Answer from the drawing. Dimensions are ordinates in mm from the lowest x, y and z of the part. A direction names the side the tool comes from. Round coordinates to 2 decimals unless told otherwise and drop trailing zeros. Write each loop counter-clockwise with the first axis right and the second up, starting at its lowest first coordinate (ties: lowest second). Pieces come first, ordered by that corner, then holes.
1. Find section A-A (y = 67.5). Write down the section's boundary in (x, z), and give its area (3 significant figures).
2. Flat-ended cylindrical pins translate along their axes: pin 1 Ø10.5 at (x, z) = (64, 18) entering from +Y; pin 2 Ø3 at (y, z) = (48.5, 44.5) entering from +X; pin 3 Ø9 at (x, z) = (10, 10) entering from +Y; pin 4 Ø10.5 at (x, y) = (14, 62) entering from -Z. Find the tip coordinate at first contact, or state that the pin passes through.
3. Find section C-C (x = 40). Write down the section's boundary in (y, z), and give its area (3 significant figures).
4. A tool of negligible diameter and unlimited length cuts with its end or side. For the marked faces 1, 2 and 3, from which of +Z, -Z, +X, -X, +Y, -Y can it reach the whole face along a straight path? Write none if from no direction.
5. Straight lines are drawn through the part: probe 1 along X at (y, z) = (7.75, 10); probe 2 along Y at (x, z) = (8.5, 52); probe 3 along X at (y, z) = (26, 41.5). For each, find the intervals that lie inside material, in ascending order.
6. Find section D-D (x = 22). Write down the section's boundary in (y, z), and give its area (3 significant figures).
7. Find section B-B (z = 26). Write down the section's boundary in (x, y), and give its area (3 significant figures).
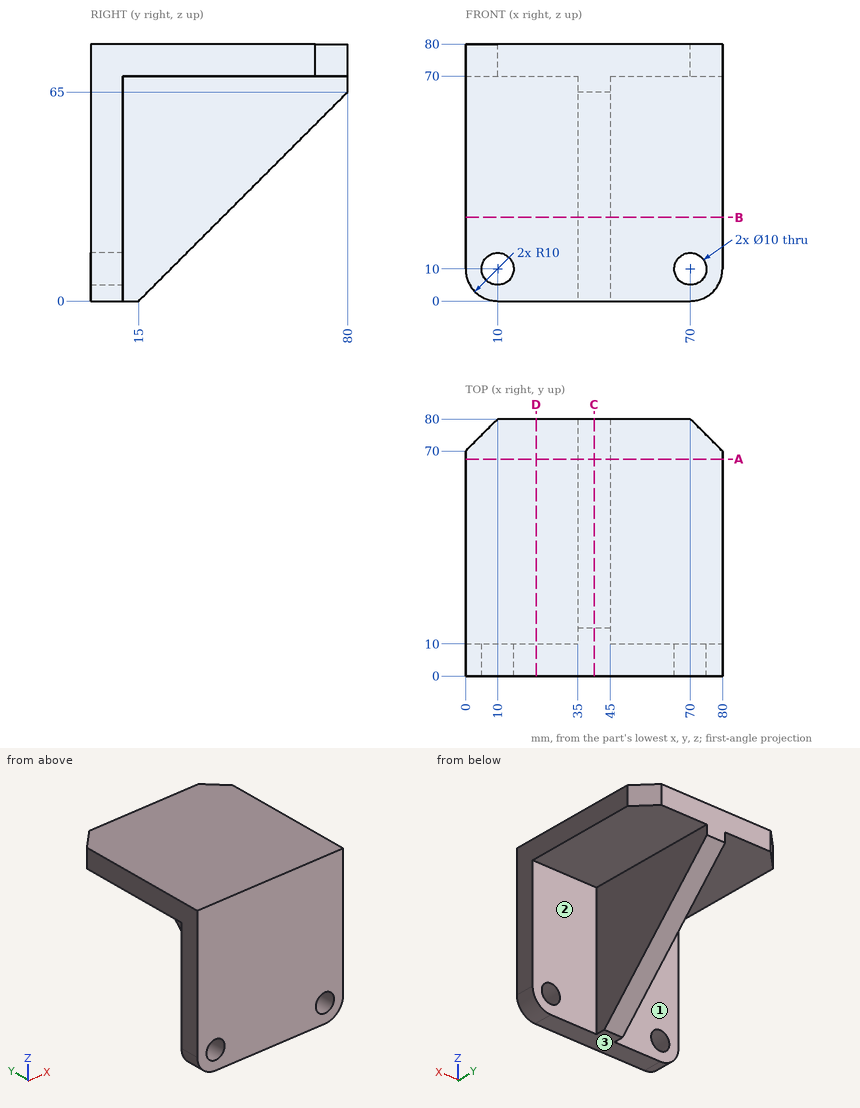
Worked answers:
1. outline: (0, 70) - (35, 70) - (35, 52.5) - (45, 52.5) - (45, 70) - (80, 70) - (80, 80) - (0, 80) - close
1. area: 975 mm2
2. pin 1: stops at y = 10
2. pin 2: stops at x = 45
2. pin 3: passes through
2. pin 4: stops at z = 70
3. outline: (0, 0) - (15, 0) - (80, 65) - (80, 80) - (0, 80) - close
3. area: 4,290 mm2
4. face 1: -Z, -X, +Y
4. face 2: -Z, +X, +Y
4. face 3: -Z, +X, -X, +Y, -Y
5. probe 1: x = 0 to 5, 15 to 65, 75 to 80
5. probe 2: y = 0 to 10
5. probe 3: x = 35 to 45
6. outline: (0, 0) - (10, 0) - (10, 70) - (80, 70) - (80, 80) - (0, 80) - close
6. area: 1,500 mm2
7. outline: (0, 0) - (80, 0) - (80, 10) - (45, 10) - (45, 41) - (35, 41) - (35, 10) - (0, 10) - close
7. area: 1,110 mm2
